Verification items for this drawing (mm, ordinates from the low corner). A direction names the side the tool comes from. Round coordinates to 2 decimals unless told otherwise and drop trailing zeros. Loops run counter-clockwise (first coordinate to the right, second up) from the corner with the lowest first, then second, coordinate; pieces in that order, holes last. Notation, with made-up numbers: (21, 74) - (48, 74) arc R10 cw to (48, 81) - close; hole circle Ø1 at (35, 69). An arc over 180 degrees is marked (long way). Put each result on its own line as item: value.
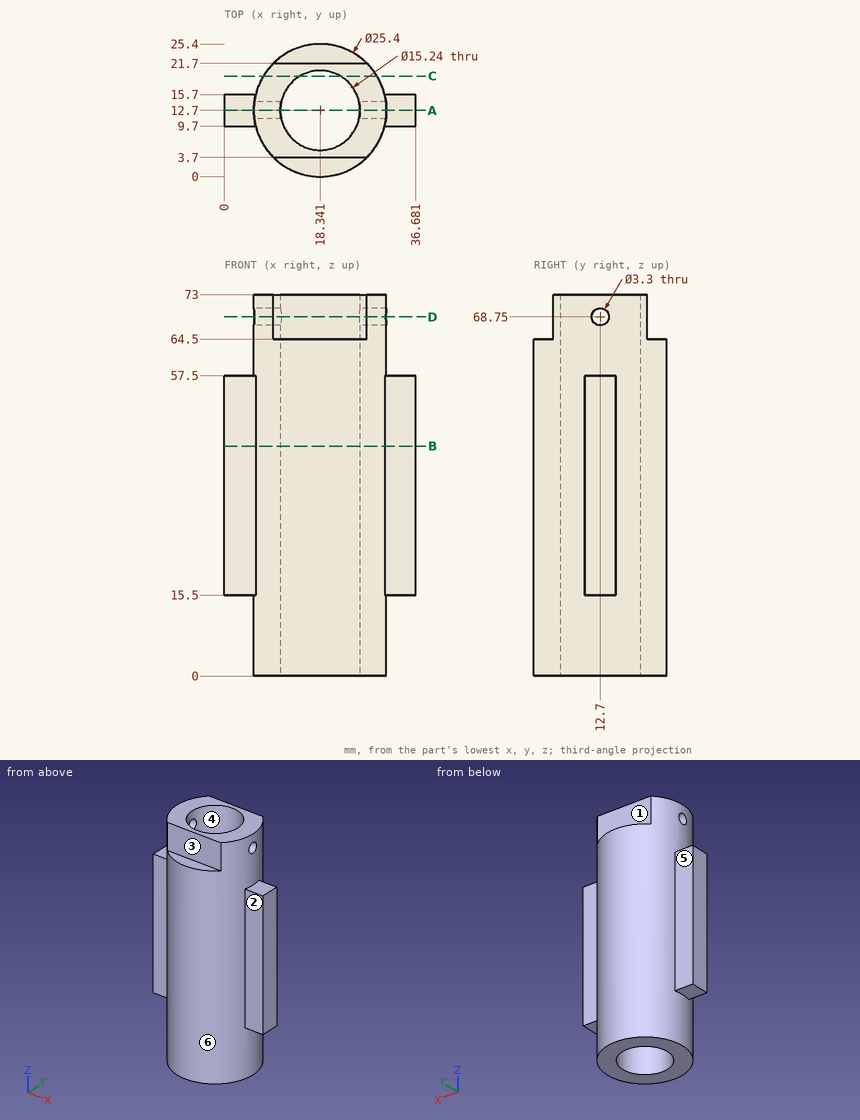
Item 1: Release check for a two-part mould opening along X. For the marked faces 4, 5 and 6 record: +X half, -X half, draft (parallel to the pull), parting line (faces both ways), or undercut.
Filled sheet:
face 4: undercut
face 5: draft
face 6: parting line
Item 2: Section check C-C on y = 19.25. Enter the section's corners in (x, z) (1 decimal).
Filled sheet:
outline: (7.5, 0) - (14.4, 0) - (14.4, 73) - (7.5, 73) - close; (22.2, 0) - (29.2, 0) - (29.2, 73) - (22.2, 73) - close
Item 3: Section check B-B on z = 44. Enter the section's corners in (x, y).
Filled sheet:
outline: (0, 9.7) - (6, 9.7) arc R12.7 ccw to (30.68, 9.7) - (36.68, 9.7) - (36.68, 15.7) - (30.68, 15.7) arc R12.7 ccw to (6, 15.7) - (0, 15.7) - close; hole circle Ø15.24 at (18.34, 12.7)
Item 4: Section check A-A on y = 12.7. Enter the section's corners in (x, z), then the cut area to 3 significant figures.
Filled sheet:
outline: (0, 15.5) - (5.64, 15.5) - (5.64, 0) - (10.72, 0) - (10.72, 67.1) - (5.64, 67.1) - (5.64, 57.5) - (0, 57.5) - close; (5.64, 70.4) - (10.72, 70.4) - (10.72, 73) - (5.64, 73) - close; (25.96, 0) - (31.04, 0) - (31.04, 15.5) - (36.68, 15.5) - (36.68, 57.5) - (31.04, 57.5) - (31.04, 67.1) - (25.96, 67.1) - close; (25.96, 70.4) - (31.04, 70.4) - (31.04, 73) - (25.96, 73) - close
area: 1,180 mm²
Item 5: Section check D-D on z = 68.75. Enter the section's corners in (x, y).
Filled sheet:
outline: (5.75, 11.05) arc R12.7 ccw to (9.38, 3.7) - (27.3, 3.7) arc R12.7 ccw to (30.93, 11.05) - (25.78, 11.05) arc R7.62 cw to (10.9, 11.05) - close; (5.75, 14.35) - (10.9, 14.35) arc R7.62 cw to (25.78, 14.35) - (30.93, 14.35) arc R12.7 ccw to (27.3, 21.7) - (9.38, 21.7) arc R12.7 ccw to start
Item 6: Tool access check on the marked faces 1, 2 and 3. Record the directions out of +Z, -Z, +X, -X, +Y, -Y that give a thin tool (end or side, any length) a straight path to the whole face; none if there is none.
Filled sheet:
face 1: +Z, +X, -X, +Y
face 2: +Z, -Z, +X, -Y
face 3: +Z, +X, -X, -Y
Item 7: Thickness scan on line 1 (Y direction, x = 18, z = 69); line 2 (X direction, y = 7.75, z = 26) (1 decimal); line 3 (Y direction, x = 14, z = 51.5) (1 decimal). Record the ranges inside material, lowest first. Write a range as from..to.
Filled sheet:
line 1: 3.7..5.09, 20.31..21.7
line 2: 6.6..12.5, 24.1..30
line 3: 0.8..6.4, 19..24.6
Item 8: Go/stop test with flat-tipped pins: pin 1 (12 mm diameter, centred on x = 22, y = 15.5, fed in from +Z); pin 2 (5 mm diameter, centred on x = 32.5, z = 30, fed in from +Y) (1 decimal); pin 3 (8 mm diameter, centred on x = 28, z = 60.5, fed in from -Y); pin 4 (8 mm diameter, centred on x = 26, z = 33, fed in from +Y). Record where each tip stops, or that it passes through.
Filled sheet:
pin 1: z = 73
pin 2: y = 17.7
pin 3: y = 1.33
pin 4: y = 24.86
